from build123d import *

# Parameters (mm, degrees)
BOSS_EXTRUDE1_DEPTH = 18.415
CUT_EXTRUDE1_DEPTH  = 12.7


with BuildPart() as part:
    # Sketch3 → Boss-Extrude1 (new body)
    with BuildSketch(Plane(origin=(0, 0, 0), x_dir=(1, 0, 0), z_dir=(0, 1, 0))):
        with BuildLine():
            Line((101.599873, 0), (110.066582, 0))
            Line((110.066582, 0), (110.066582, 42.333418))
            Line((110.066582, 42.333418), (55.033291, 42.333418))
            Line((55.033291, 42.333418), (8.4666328, 42.333418))
            Line((8.4666328, 42.333418), (0, 42.333418))
            Line((0, 42.333418), (0, 0))
            Line((0, 0), (8.4666328, 0))
            Line((8.4666328, 0), (8.4666328, -25.4))
            Line((8.4666328, -25.4), (12.6999492, -35.56))
            Line((12.6999492, -35.56), (12.6999492, -69.426582))
            add(Edge.make_bspline(
                [(12.6999492, -69.426582), (11.690404189, -80.766544706), (8.46666328, -91.44)],
                knots=[0, 0, 0, 0.504540069, 0.504540069, 0.504540069], degree=2))
            Line((8.46666328, -91.44), (8.46666328, -111.76))
            Line((8.46666328, -111.76), (101.599995682, -111.76))
            Line((101.599995682, -111.76), (101.599995682, -91.44))
            add(Edge.make_bspline(
                [(97.366709, -69.426582), (98.376270675, -80.766537876), (101.599995682, -91.44)],
                knots=[0, 0, 0, 0.504540407, 0.504540407, 0.504540407], degree=2))
            Line((97.366709, -69.426582), (97.366709, -35.56))
            Line((97.366709, -35.56), (101.599873, -25.4))
            Line((101.599873, -25.4), (101.599873, 0))
        make_face()
    extrude(amount=BOSS_EXTRUDE1_DEPTH)

    # Sketch7 → Cut-Extrude1 (cut)
    with BuildSketch(Plane(origin=(0, 18.415, 0), x_dir=(1, 0, 0), z_dir=(0, 1, 0))):
        with BuildLine():
            Line((104.986582, 5.08), (104.986582, 37.253418))
            Line((104.986582, 37.253418), (5.08, 37.253418))
            Line((5.08, 37.253418), (5.08, 5.08))
            Line((5.08, 5.08), (13.5466328, 5.08))
            Line((13.5466328, 5.08), (13.5466328, -24.384003751))
            Line((13.5466328, -24.384003751), (17.7799492, -34.544003751))
            Line((17.7799492, -34.544003751), (17.7799492, -69.649806794))
            add(Edge.make_bspline(
                [(13.54666328, -92.18157962), (15.696718758, -84.885689198), (17.107633166, -77.368389863), (17.7799492, -69.649806794)],
                knots=[0, 0, 0, 0, 1, 1, 1, 1], degree=3))
            Line((13.54666328, -92.18157962), (13.54666328, -106.68))
            Line((13.54666328, -106.68), (96.519995682, -106.68))
            Line((96.519995682, -106.68), (96.519995682, -92.1815758))
            add(Edge.make_bspline(
                [(92.286709, -69.649810631), (92.959036165, -77.368387225), (94.369950858, -84.885683715), (96.519995682, -92.1815758)],
                knots=[0, 0, 0, 0, 1, 1, 1, 1], degree=3))
            Line((92.286709, -69.649810631), (92.286709, -34.544037514))
            Line((92.286709, -34.544037514), (96.519873, -24.384037514))
            Line((96.519873, -24.384037514), (96.519873, 5.08))
            Line((96.519873, 5.08), (104.986582, 5.08))
        make_face()
    extrude(amount=-CUT_EXTRUDE1_DEPTH, mode=Mode.SUBTRACT)


solid = part.part
Design review of the part built by this model. Coordinates are the model's own, in mm. A direction names the side the tool comes from. Round coordinates to 2 decimals unless told otherwise and drop trailing zeros. Write each loop counter-clockwise with the first axis right and the second up, starting at its lowest first coordinate (ties: lowest second). Pieces come first, ordered by that corner, then holes. Notation, with made-up numbers: M -27.5,55 L 24.5,55 A28 cw 24.5,91 Z; hole C 36.5,6.5 d7. An arc over 180 degrees is marked long. One line per item, written item: value. Start each with the question number.
1. Take a section at B-B on z = 57.5. State the section outline as (x, y) points (3 decimals).
2. For faces 1 (the face through (8.467, 9, 101)), 2 (the face through (101, 12, -5.08)), 3 (the face through (99.454, 9.079, 30.551)), 4 (the face through (101.6, 9, 102)), 5 (the face through (10.554, 9.079, 30.409)), list the 3-axis set-ups (+Z, -Z, +X, -X, +Y, -Y) from which the entire face can be reached by the end or side of a thin tool; tool diameter is ignored.
3. Clearance check with flat-ended pins moving along their axes: P1, Ø4, axis at x = 24.5, z = 92.5, coming from the -Y side; P2, Ø10, axis at y = 14, z = 50, coming from the -X side; P3, Ø1, axis at y = 6, z = 69, coming from the +X side; P4, Ø9, axis at y = 10.5, z = 13, coming from the +X side. State where each tip first meets the part, or that it passes through.
4. Take a section at A-A on x = 90.5. State the section outline as (y, z) points (3 decimals), then the cut area to 3 significant figures.
5. To check wall thickness, follow probe 1 along X at (y, z) = (12.25, 46); probe 2 along Z at (x, y) = (19, 7.25); probe 3 along X at (y, z) = (13, 8.5). State the ranges of each line that lie inside material, in increasing order. Write a range as from..to.
Computed:
1. outline: M 12.7,0 L 97.367,0 L 97.367,18.415 L 92.287,18.415 L 92.287,5.715 L 17.78,5.715 L 17.78,18.415 L 12.7,18.415 Z
2. face 1: +Z, -X, +Y, -Y
2. face 2: +Y
2. face 3: +X, +Y, -Y
2. face 4: +Z, +X, +Y, -Y
2. face 5: -X, +Y, -Y
3. P1: stops at y = 0
3. P2: stops at x = 12.7
3. P3: stops at x = 97.37
3. P4: stops at x = 101.6
4. outline: M 0,-42.333 L 18.415,-42.333 L 18.415,-37.253 L 5.715,-37.253 L 5.715,106.68 L 18.415,106.68 L 18.415,111.76 L 0,111.76 Z
4. area: 1,010 mm²
5. probe 1: x = 12.7..17.78, 92.29..97.37
5. probe 2: z = -42.33..-37.25, 106.68..111.76
5. probe 3: x = 8.47..13.55, 96.52..101.6
